Answer from the drawing. Dimensions are ordinates in mm from the lowest x, y and z of the part. A direction names the side the tool comes from. Give positions to 0.01 mm unless a question says otherwise; leave off trailing zeros. Order: outer loops, then holes, each group sorted by start corner. A loop starts at its lowest first (then second) coordinate and runs counter-clockwise, first axis right, second up. Notation, with made-up numbers: (55, -37.5) - (74, -37.5) arc R13 ccw to (74, -27.5) - close; hole circle Ø6 at (-39.5, -7). An arc over 180 degrees is marked (long way). Use a Markdown table: item, result. Add a question column.
1) Find section C-C, the plane x = 12.75. Determine the outline of the cut face in (y, z), plus the area to 3 significant figures.
2) A flat-ended cylindrical pin translates along its axis: pin 1 (0.6 mm diameter, centred on y = 7, z = 0.5, fed in from -X). Find the tip coordinate at first contact, or state that the pin passes through.
3) Find section D-D, the plane y = 6. Determine the outline of the cut face in (x, z), plus the area to 4 significant figures.
4) Straight lines are drawn through the part: line 1 (X direction, y = 7, z = 1.2); line 2 (X direction, y = 5, z = 0.2); line 3 (Y direction, x = 1, z = 0.65). For each, find the intervals that lie inside material, in ascending order.
5) Find section A-A, the plane z = 0.65. Determine the outline of the cut face in (x, y).
6) The mould has two halves that part along Y. Classify the marked faces 4, 5, 6 and 7: released by +Y, released by -Y, zero draft, split by the parting line, or undercut.
7) Find section B-B, the plane y = 8.75. Determine the outline of the cut face in (x, z), plus the area to 3 significant figures.
8) For the marked faces 1, 2 and 3, determine the directions among +Z, -Z, +X, -X, +Y, -Y from which every point of the face is accessible in a straight line to the end or side of a thin tool.
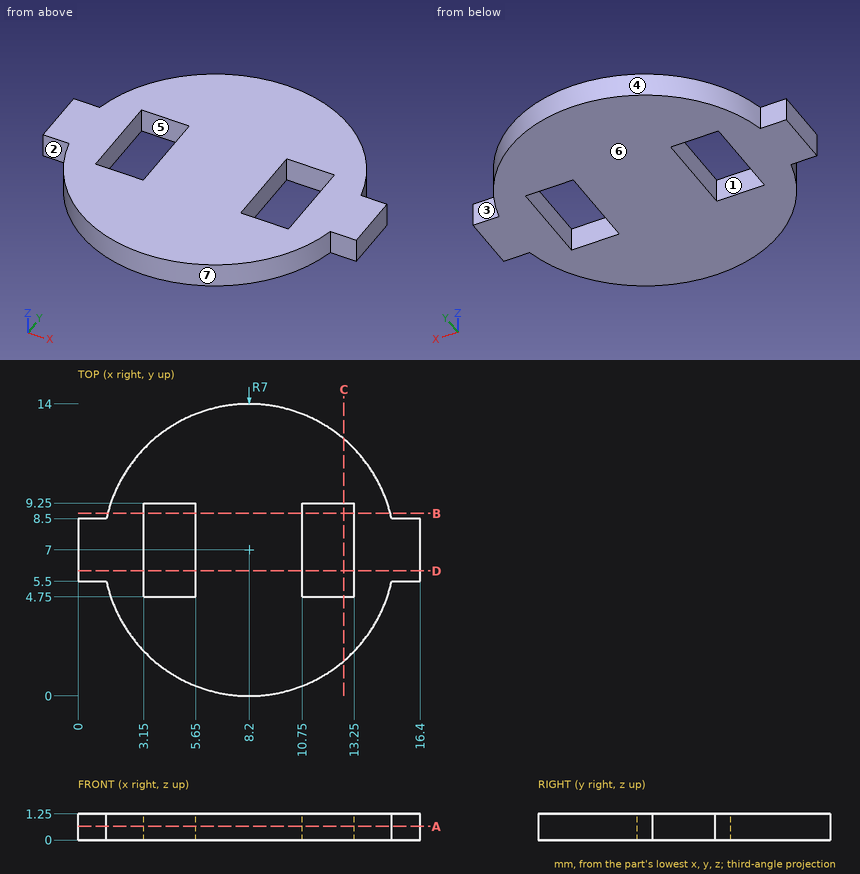
The answers:
| question | item | result |
|---|---|---|
| 1 | outline | (1.68, 0) - (4.75, 0) - (4.75, 1.25) - (1.68, 1.25) - close; (9.25, 0) - (12.32, 0) - (12.32, 1.25) - (9.25, 1.25) - close |
| 1 | area | 7.67 mm2 |
| 2 | pin 1 | x = 0 |
| 3 | outline | (0, 0) - (3.15, 0) - (3.15, 1.25) - (0, 1.25) - close; (5.65, 0) - (10.75, 0) - (10.75, 1.25) - (5.65, 1.25) - close; (13.25, 0) - (16.4, 0) - (16.4, 1.25) - (13.25, 1.25) - close |
| 3 | area | 14.25 mm2 |
| 4 | line 1 | 0 to 3.15, 5.65 to 10.75, 13.25 to 16.4 |
| 4 | line 2 | 1.49 to 3.15, 5.65 to 10.75, 13.25 to 14.91 |
| 4 | line 3 | 5.5 to 8.5 |
| 5 | outline | (0, 5.5) - (1.36, 5.5) arc R7 ccw to (15.04, 5.5) - (16.4, 5.5) - (16.4, 8.5) - (15.04, 8.5) arc R7 ccw to (1.36, 8.5) - (0, 8.5) - close; hole (3.15, 4.75) - (5.65, 4.75) - (5.65, 9.25) - (3.15, 9.25) - close; hole (10.75, 4.75) - (13.25, 4.75) - (13.25, 9.25) - (10.75, 9.25) - close |
| 6 | face 4 | released by +Y |
| 6 | face 5 | undercut |
| 6 | face 6 | zero draft |
| 6 | face 7 | released by -Y |
| 7 | outline | (1.42, 0) - (3.15, 0) - (3.15, 1.25) - (1.42, 1.25) - close; (5.65, 0) - (10.75, 0) - (10.75, 1.25) - (5.65, 1.25) - close; (13.25, 0) - (14.98, 0) - (14.98, 1.25) - (13.25, 1.25) - close |
| 7 | area | 10.7 mm2 |
| 8 | face 1 | +Z, -Z |
| 8 | face 2 | +Z, -Z, -X, -Y |
| 8 | face 3 | +Z, -Z, +X, +Y |
